Can you work these out from the model? Positions are in its coordinate system, mm. A direction names the side the tool comes from. Coordinates: 2 decimals unless noted, no trailing zeros. Write each loop counter-clockwise with the first axis right and the second up, starting at its lowest first coordinate (ties: lowest second). Pieces come first, ordered by that corner, then holes. Notation, with made-up numbers: (49.5, 41.25) - (86.5, 41.25) arc R16 ccw to (86.5, 55.25) - close; hole circle Ø7 at (42.5, -4.75). An arc over 180 degrees is marked (long way). Use one line per item in the form item = value. Start each with the question number.
(1) If we section it at B-B on z = 741.5: Please give me the cut outline in (x, y).
(2) If I drill on probe 1 along Y at (x, z) = (136.5, 356); probe 2 along X at (y, z) = (480, 58); probe 3 along X at (y, z) = (250.5, 719), over which ranges is the centre line in solid material (lowest first)? Write a range as from..to.
(3) On a 3-axis mill with a long thin cutter (end or side, diameter ignored), from which of +Z, -Z, +X, -X, +Y, -Y can I reach the whole of each face in a straight line? I mean faces 1 (the face through (-5, 527.05, 626)), 2 (the face through (5, 539.75, 626)). Say none if no direction works.
(4) If we section it at C-C on y = 159: Please give me the cut outline in (x, z).
(5) Thinking about a two-plate mould opening in Y: for faces 3 (the face through (-403.824, 525.264, 626.11)), 4 (the face through (6, 6.35, 626)), 5 (the face through (419.1, 238, 626)), which applies, pulls with the +Y half, pulls with the -Y half, needs draft (parallel to the pull), parting line crosses it, or undercut?
(6) For pin 1 Ø10 at (x, z) = (-414.5, 845) entering from +Y; pin 2 Ø10 at (y, z) = (161, 267.5) entering from -X, each with a flat end and sliding along its axis, tell me the tip position at first contact or that it passes through.
(7) If we section it at A-A on x = 243.5: Please give me the cut outline in (y, z).
```python
from build123d import *

# Parameters (mm, degrees)
F0_W     = 12.7
F0_H     = 25.4
F1_DEPTH = 1270


with BuildPart() as f1:
    # F0 (on Top) → F1 (new body)
    with BuildSketch(Plane.XY):
        with Locations((-412.75, 19.05)):
            Rectangle(F0_W, F0_H)
        Polygon((-406.4, 6.35), (-419.1, 6.35), (-419.1, -6.35), (419.1, -6.35), (419.1, 6.35), (406.4, 6.35), align=None)
        with BuildLine():
            Line((406.4, 476.25), (406.4, 6.35))
            Line((406.4, 6.35), (419.1, 6.35))
            Line((419.1, 6.35), (419.1, 488.95))
            ThreePointArc((419.1, 488.95), (404.221024, 524.871024), (368.3, 539.75))
            Line((368.3, 539.75), (-368.3, 539.75))
            ThreePointArc((-368.3, 539.75), (-404.221024, 524.871024), (-419.1, 488.95))
            Line((-419.1, 488.95), (-419.1, 476.25))
            Line((-419.1, 476.25), (-406.4, 476.25))
            ThreePointArc((-406.4, 476.25), (-391.521024, 512.171024), (-355.6, 527.05))
            Line((-355.6, 527.05), (355.6, 527.05))
            ThreePointArc((355.6, 527.05), (391.521024, 512.171024), (406.4, 476.25))
        make_face()
    extrude(amount=F1_DEPTH)


solid = f1.part
```
Reported:
q1.outline = (-419.1, -6.35) - (419.1, -6.35) - (419.1, 488.95) arc R50.8 ccw to (368.3, 539.75) - (-368.3, 539.75) arc R50.8 ccw to (-419.1, 488.95) - (-419.1, 476.25) - (-406.4, 476.25) arc R50.8 cw to (-355.6, 527.05) - (355.6, 527.05) arc R50.8 cw to (406.4, 476.25) - (406.4, 6.35) - (-406.4, 6.35) - (-406.4, 31.75) - (-419.1, 31.75) - close
q2.probe_1 = -6.35..6.35, 527.05..539.75
q2.probe_2 = -419.1..-406.26, 406.26..419.1
q2.probe_3 = 406.4..419.1
q3.face_1 = +Z, -Z
q3.face_2 = +Z, -Z, +X, -X, +Y
q4.outline = (406.4, 0) - (419.1, 0) - (419.1, 1270) - (406.4, 1270) - close
q5.face_3 = pulls with the +Y half
q5.face_4 = undercut
q5.face_5 = needs draft
q6.pin_1 = 518.67
q6.pin_2 = 406.4
q7.outline = (-6.35, 0) - (6.35, 0) - (6.35, 1270) - (-6.35, 1270) - close; (527.05, 0) - (539.75, 0) - (539.75, 1270) - (527.05, 1270) - close
